Input: part model. Units: mm. Frame: model coordinates. Face numbers are marked on the shaded views. A direction names the side the tool comes from. Give positions to 0.01 mm unless a question says otherwise; leave off trailing zeros. Loops run counter-clockwise (first coordinate to the right, second up) from the corner with the lowest first, then second, coordinate; pieces in that order, holes last. Notation, with made-up numbers: M 28.5,2 L 56.5,2 A12 cw 56.5,11 Z; hole C 30.5,3 d4. An arc over 180 degrees is marked long. Use a Markdown table: item, result. Add a question column.
from build123d import *

# Parameters (mm, degrees)
ESTRUSIONE_ESTRUSIONE1_DEPTH          = 3
FORO_SVASATO_PER_VITE_M4_1_AT_2_COUNT = 2
FORO_SVASATO_PER_VITE_M4_1_AT_2_PITCH = 95
FORO_SVASATO_PER_VITE_M3_1_AT_2_COUNT = 2
FORO_SVASATO_PER_VITE_M3_1_AT_2_PITCH = 60.5
FORO_SVASATO_PER_VITE_M3_1_AT_3_COUNT = 2
FORO_SVASATO_PER_VITE_M3_1_AT_3_PITCH = 88.782036471
FORO_SVASATO_PER_VITE_M3_1_AT_4_COUNT = 2
FORO_SVASATO_PER_VITE_M3_1_AT_4_PITCH = 38.5
TAGLIO_ESTRUSIONE2_REACH              = 73.691
SCHIZZO9_R                            = 1.75
SKETCH4_W                             = 25
SKETCH4_H                             = 10
BOSS_EXTRUDE3_DEPTH                   = 30
SKETCH6_R                             = 3
CUT_EXTRUDE2_DEPTH                    = 111.474544579
CHAMFER1_SIZE                         = 2
FILLET1_R                             = 10


with BuildPart() as part:
    # Schizzo1 → Estrusione-Estrusione1 (new body)
    with BuildSketch(Plane.XY):
        with BuildLine():
            Line((20.25, -47.5), (23.25, -47.5))
            Line((23.25, -47.5), (23.25, 47.5))
            Line((23.25, 47.5), (20.25, 47.5))
            ThreePointArc((20.25, 47.5), (0, 67.75), (-20.25, 47.5))
            Line((-20.25, 47.5), (-23.25, 47.5))
            Line((-23.25, 47.5), (-23.25, -47.5))
            Line((-23.25, -47.5), (-20.25, -47.5))
            ThreePointArc((-20.25, -47.5), (0, -67.75), (20.25, -47.5))
        make_face()
    extrude(amount=ESTRUSIONE_ESTRUSIONE1_DEPTH)

    # Schizzo5 → Foro svasato per Vite M4-1 (revolve, cut)
    with BuildSketch(Plane(origin=(0, 47.5, 0), x_dir=(0, 1, 0), z_dir=(1, 0, 0))):
        Polygon((0, 0), (0, 3), (2.25, 3), (2.25, 2.45), (4.7, 0), align=None)
    foro_svasato_per_vite_m4_1 = revolve(axis=Axis((0, 47.5, -6.35), (0, 0, 1)), mode=Mode.SUBTRACT)

    # Foro svasato per Vite M4-1 at 2: Foro svasato per Vite M4-1 ×2
    with Locations(*[(0, -i * FORO_SVASATO_PER_VITE_M4_1_AT_2_PITCH, 0) for i in range(1, FORO_SVASATO_PER_VITE_M4_1_AT_2_COUNT)]):
        add(foro_svasato_per_vite_m4_1, mode=Mode.SUBTRACT)

    # Schizzo8 → Foro svasato per Vite M3-1 (revolve, cut)
    with BuildSketch(Plane(origin=(19.25, 40, 0), x_dir=(0, 1, 0), z_dir=(1, 0, 0))):
        Polygon((0, 0), (0, 3), (1.7, 3), (1.7, 1.45), (3.15, 0), align=None)
    foro_svasato_per_vite_m3_1 = revolve(axis=Axis((19.25, 40, -6.35), (0, 0, 1)), mode=Mode.SUBTRACT)

    # Foro svasato per Vite M3-1 at 2: Foro svasato per Vite M3-1 ×2
    with Locations(*[(0, -i * FORO_SVASATO_PER_VITE_M3_1_AT_2_PITCH, 0) for i in range(1, FORO_SVASATO_PER_VITE_M3_1_AT_2_COUNT)]):
        add(foro_svasato_per_vite_m3_1, mode=Mode.SUBTRACT)

    # Foro svasato per Vite M3-1 at 3: Foro svasato per Vite M3-1 ×2
    with Locations(*[Vector(-0.43364628172754605, -0.9010831828104849, 0) * (i * FORO_SVASATO_PER_VITE_M3_1_AT_3_PITCH) for i in range(1, FORO_SVASATO_PER_VITE_M3_1_AT_3_COUNT)]):
        add(foro_svasato_per_vite_m3_1, mode=Mode.SUBTRACT)

    # Foro svasato per Vite M3-1 at 4: Foro svasato per Vite M3-1 ×2
    with Locations(*[(-i * FORO_SVASATO_PER_VITE_M3_1_AT_4_PITCH, 0, 0) for i in range(1, FORO_SVASATO_PER_VITE_M3_1_AT_4_COUNT)]):
        add(foro_svasato_per_vite_m3_1, mode=Mode.SUBTRACT)

    # Schizzo9 → Taglio-Estrusione2 (cut, up to next)
    with BuildSketch(Plane(origin=(0, 0, 0), x_dir=(-1, 0, 0), z_dir=(0, 0, -1)), mode=Mode.PRIVATE) as taglio_estrusione2_sk1:
        with Locations((-19.25, 0)):
            Circle(SCHIZZO9_R)
    taglio_estrusione2_tool1 = extrude(taglio_estrusione2_sk1.sketch, amount=-TAGLIO_ESTRUSIONE2_REACH, mode=Mode.PRIVATE) & part.part
    # Schizzo9 → Taglio-Estrusione2 (cut, up to next)
    with BuildSketch(Plane(origin=(0, 0, 0), x_dir=(-1, 0, 0), z_dir=(0, 0, -1)), mode=Mode.PRIVATE) as taglio_estrusione2_sk2:
        with Locations((19.25, 0)):
            Circle(SCHIZZO9_R)
    taglio_estrusione2_tool2 = extrude(taglio_estrusione2_sk2.sketch, amount=-TAGLIO_ESTRUSIONE2_REACH, mode=Mode.PRIVATE) & part.part
    # Schizzo9 → Taglio-Estrusione2 (cut, up to next)
    with BuildSketch(Plane(origin=(0, 0, 0), x_dir=(-1, 0, 0), z_dir=(0, 0, -1)), mode=Mode.PRIVATE) as taglio_estrusione2_sk3:
        with Locations((0, 65.25)):
            Circle(SCHIZZO9_R)
    taglio_estrusione2_tool3 = extrude(taglio_estrusione2_sk3.sketch, amount=-TAGLIO_ESTRUSIONE2_REACH, mode=Mode.PRIVATE) & part.part
    # Schizzo9 → Taglio-Estrusione2 (cut, up to next)
    with BuildSketch(Plane(origin=(0, 0, 0), x_dir=(-1, 0, 0), z_dir=(0, 0, -1)), mode=Mode.PRIVATE) as taglio_estrusione2_sk4:
        with Locations((0, -65.25)):
            Circle(SCHIZZO9_R)
    taglio_estrusione2_tool4 = extrude(taglio_estrusione2_sk4.sketch, amount=-TAGLIO_ESTRUSIONE2_REACH, mode=Mode.PRIVATE) & part.part
    add(taglio_estrusione2_tool1.solids().sort_by_distance((19.25, 0, 0))[0], mode=Mode.SUBTRACT)
    add(taglio_estrusione2_tool2.solids().sort_by_distance((-19.25, 0, 0))[0], mode=Mode.SUBTRACT)
    add(taglio_estrusione2_tool3.solids().sort_by_distance((0, 65.25, 0))[0], mode=Mode.SUBTRACT)
    add(taglio_estrusione2_tool4.solids().sort_by_distance((0, -65.25, 0))[0], mode=Mode.SUBTRACT)

    # Sketch4 → Boss-Extrude3 (add)
    with BuildSketch(Plane(origin=(0, 0, 0), x_dir=(-1, 0, 0), z_dir=(0, 0, -1))):
        with Locations((0, 31)):
            Rectangle(SKETCH4_W, SKETCH4_H)
        with Locations((0, -31)):
            Rectangle(SKETCH4_W, SKETCH4_H)
    extrude(amount=BOSS_EXTRUDE3_DEPTH)

    # Sketch6 → Cut-Extrude2 (cut, through all)
    with BuildSketch(Plane(origin=(0, 36, 0), x_dir=(1, 0, 0), z_dir=(0, 1, 0))):
        with Locations(Location((0, 15, 0), (0, 0, 180))):
            Circle(SKETCH6_R)
    extrude(amount=-CUT_EXTRUDE2_DEPTH, mode=Mode.SUBTRACT)

    # Chamfer1
    chamfer1_edges = [part.edges().sort_by_distance(p)[0] for p in [
        (-12.5, 31, 0),
        (0, 36, 0),
        (12.5, 31, 0),
        (0, 26, 0),
        (0, -26, 0),
        (12.5, -31, 0),
        (0, -36, 0),
        (-12.5, -31, 0),
    ]]
    chamfer(chamfer1_edges, length=CHAMFER1_SIZE)

    # Fillet1
    fillet1_edges = [part.edges().sort_by_distance(p)[0] for p in [
        (-12.5, -31, -30),
        (-12.5, 31, -30),
        (12.5, 31, -30),
        (12.5, -31, -30),
    ]]
    fillet(fillet1_edges, radius=FILLET1_R)


solid = part.part
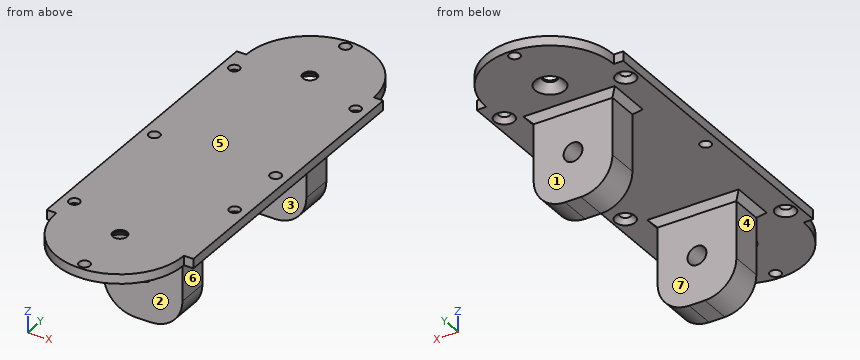
1) Section query A-A, the plane y = 0. Return the cut outline in (x, z).
2) Pull-direction query (Y, two-part tool) for the marked faces 1, 2 and 3; classes: pulls with the +Y half, pulls with the -Y half, needs draft (parallel to the pull), parting line crosses it, or undercut.
3) Section query C-C, the plane y = -40. Return the cut outline in (x, z).
4) Reachability of the marked faces 4, 5, 6 and 7 from +Z, -Z, +X, -X, +Y, -Y: full face, straight path, thin tool, end or side. Return the list, or none.
5) Contact query for flat-ended pins moving along their axis: P1, Ø3, axis at x = -6, z = -9.5, coming from the -Y side; P2, Ø4, axis at x = -14.5, z = -22.5, coming from the -Y side; P3, Ø12.5, axis at x = 2.5, z = -17, coming from the +Y side; P4, Ø4.5, axis at x = -19.25, y = 0, coming from the -Z side. Output: stop coordinate, or through.
6) Section query D-D, the plane z = -15. Return the cut outline in (x, y).
7) Section query B-B, the plane z = -6. Return the cut outline in (x, y), and give its area (3 significant figures).
8) Ray query, line 1 (Y direction, x = 0, z = 2.9); line 2 (Z direction, x = 0, y = -32.5); line 3 (Y direction, x = 10.5, z = -24). Return the intervals inside material, ascending. Write a range as [from, to].
Entries:
| question | item | result |
|---|---|---|
| 1 | outline | M -23.25,0 L -21,0 L -21,3 L -23.25,3 Z; M -17.5,0 L 17.5,0 L 17.5,3 L -17.5,3 Z; M 21,0 L 23.25,0 L 23.25,3 L 21,3 Z |
| 2 | face 1 | pulls with the +Y half |
| 2 | face 2 | pulls with the -Y half |
| 2 | face 3 | undercut |
| 3 | outline | M -23.25,0 L -22.4,0 L -20.95,1.45 L -20.95,3 L -23.25,3 Z; M -17.55,1.45 L -16.1,0 L 23.25,0 L 23.25,3 L -17.55,3 Z |
| 4 | face 4 | -Z, -X, +Y, -Y |
| 4 | face 5 | +Z, +X, -X, +Y, -Y |
| 4 | face 6 | -Z, +X, +Y, -Y |
| 4 | face 7 | -Z, +X, -X |
| 5 | P1 | stops at y = -36 |
| 5 | P2 | passes through |
| 5 | P3 | stops at y = 36 |
| 5 | P4 | stops at z = 0 |
| 6 | outline | M -12.5,-36 L -3,-36 L -3,-26 L -12.5,-26 Z; M -12.5,26 L -3,26 L -3,36 L -12.5,36 Z; M 3,-36 L 12.5,-36 L 12.5,-26 L 3,-26 Z; M 3,26 L 12.5,26 L 12.5,36 L 3,36 Z |
| 7 | outline | M -12.5,-36 L 12.5,-36 L 12.5,-26 L -12.5,-26 Z; M -12.5,26 L 12.5,26 L 12.5,36 L -12.5,36 Z |
| 7 | area | 500 mm² |
| 8 | line 1 | y = [-67.75, -67], [-63.5, -49.75], [-45.25, 45.25], [49.75, 63.5], [67, 67.75] |
| 8 | line 2 | z = [-30, -18], [-12, 3] |
| 8 | line 3 | y = [-36, -26], [26, 36] |
